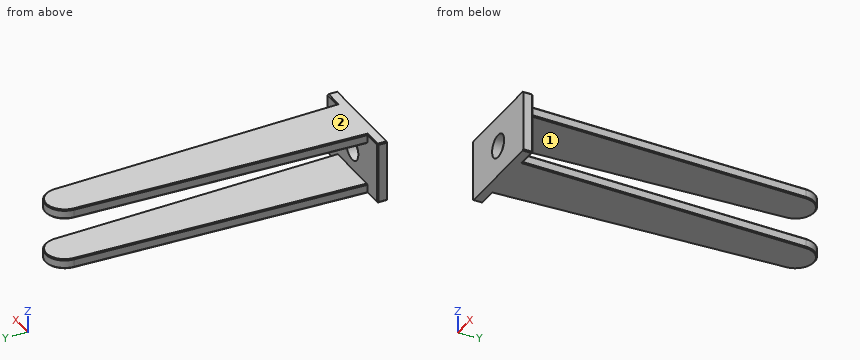
from build123d import *

# Parameters (mm, degrees)
BOSS_EXTRUDE2_DEPTH = 5
BOSS_EXTRUDE3_DEPTH = 5
SKETCH3_R           = 6
CUT_EXTRUDE1_DEPTH  = 173.768631412
CHAMFER1_SIZE       = 0.5


with BuildPart() as part:
    # Sketch2 → Boss-Extrude2 (new body)
    with BuildSketch(Plane(origin=(0, 0, 0), x_dir=(1, 0, 0), z_dir=(0, 1, 0))):
        Polygon((0, 0), (-40, 0), (-40, -16), (0, -16), (10, -16), (10, 0), align=None)
    extrude(amount=-BOSS_EXTRUDE2_DEPTH)

    # Sketch1 → Boss-Extrude3 (add)
    with BuildSketch(Plane.XY):
        with BuildLine():
            Line((0, 0), (-30, 0))
            Line((-30, 0), (-24.994461357, 150.332779469))
            ThreePointArc((-24.994461357, 150.332779469), (-15, 160), (-5.005538643, 150.332779469))
            Line((-5.005538643, 150.332779469), (0, 0))
        make_face()
    extrude(amount=BOSS_EXTRUDE3_DEPTH)

    # Mirror1: part across plane


with BuildPart() as part_1:
    add(part.part)
    add(part.part.mirror(Plane(origin=(10, -5, 16), x_dir=(1, 0, 0), z_dir=(0, 0, 1))))

    # Sketch3 → Cut-Extrude1 (cut, through all)
    with BuildSketch(Plane.XZ.offset(5)):
        with Locations(Location((-15, 16, 0), (0, 0, 270))):
            Circle(SKETCH3_R)
    extrude(amount=-CUT_EXTRUDE1_DEPTH, mode=Mode.SUBTRACT)

    # Chamfer1
    chamfer1_edges = [part_1.edges().sort_by_distance(p)[0] for p in [
        (10, -2.5, 0),
        (-40, -2.5, 0),
        (-35, 0, 0),
        (-2.502769321, 75.166389735, 0),
        (-15, 160, 0),
        (-27.497230679, 75.166389735, 0),
        (-2.502769321, 75.166389735, 5),
        (-15, 160, 5),
        (-27.497230679, 75.166389735, 5),
        (-40, -2.5, 32),
        (5, 0, 32),
        (-2.502769321, 75.166389735, 32),
        (-15, 160, 32),
        (-27.497230679, 75.166389735, 32),
        (-35, 0, 32),
        (10, -2.5, 32),
        (-2.502769321, 75.166389735, 27),
        (-15, 160, 27),
        (-27.497230679, 75.166389735, 27),
        (10, 0, 16),
        (-40, 0, 16),
        (5, 0, 0),
    ]]
    chamfer(chamfer1_edges, length=CHAMFER1_SIZE)


solid = part_1.part
Could you check a few things on this model? Use its own coordinates, in mm. Face numbers are marked on the shaded views. A direction names the side the tool comes from. Give positions to 0.01 mm unless a question says otherwise; leave off trailing zeros. Order: outer loops, then holes, each group sorted by start corner. A loop starts at its lowest first (then second) coordinate and runs counter-clockwise, first axis right, second up.
1. For pin 1 (15.5 mm diameter, centred on x = -15, z = 16, fed in from +Y); pin 2 (2 mm diameter, centred on x = 0, y = 24, fed in from +Z), each with a flat end and sliding along its axis, tell me the tip position at first contact or that it passes through.
Answers below:
pin 1: stops at y = 0
pin 2: stops at z = 31.7
2. Suppose I cut it at A-A (z = 16). Write out the boundary of the cut face in (x, y), plus the area to 3 significant figures.
Answers below:
outline: (-40, -5) - (-21, -5) - (-21, 0) - (-39.5, 0) - (-40, -0.5) - close; (-9, -5) - (10, -5) - (10, -0.5) - (9.5, 0) - (-9, 0) - close
area: 190 mm2
3. Suppose I cut it at B-B (x = -15). Write out the boundary of the cut face in (y, z), plus the area to 3 significant figures.
Answers below:
outline: (-5, 0) - (159.5, 0) - (160, 0.5) - (160, 4.5) - (159.5, 5) - (0, 5) - (0, 10) - (-5, 10) - close; (-5, 22) - (0, 22) - (0, 27) - (159.5, 27) - (160, 27.5) - (160, 31.5) - (159.5, 32) - (-5, 32) - close
area: 1,700 mm2
4. Suppose I cut it at C-C (y = 126). Write out the boundary of the cut face in (x, z).
Answers below:
outline: (-25.8, 0.5) - (-25.3, 0) - (-4.7, 0) - (-4.2, 0.5) - (-4.2, 4.5) - (-4.7, 5) - (-25.3, 5) - (-25.8, 4.5) - close; (-25.8, 27.5) - (-25.3, 27) - (-4.7, 27) - (-4.2, 27.5) - (-4.2, 31.5) - (-4.7, 32) - (-25.3, 32) - (-25.8, 31.5) - close
5. Suppose I cut it at D-D (x = -34). Write out the boundary of the cut face in (y, z), plus the area to 3 significant figures.
Answers below:
outline: (-5, 0) - (-0.5, 0) - (0, 0.5) - (0, 31.5) - (-0.5, 32) - (-5, 32) - close
area: 160 mm2
6. I need wall thicknesses on L1, parallel to X at y = -2.6, z = 16; L2, parallel to Z at x = -7, y = 84; L3, parallel to Y at x = -6, z = 21.5. Which ranges of each line are inside material? Lowest first, please.
Answers below:
L1: x = -40 to -21, -9 to 10
L2: z = 0 to 5, 27 to 32
L3: y = -5 to 0
7. Which directions (+Z, -Z, +X, -X, +Y, -Y) give clear straight access to the entire face, cutting with the end or side of a thin tool? Please do the marked faces 1 and 2.
Answers below:
face 1: +X, -X, +Y
face 2: +Z, +X, -X, +Y, -Y
